Part model, mm, in its own coordinate system. A direction names the side the tool comes from. Round coordinates to 2 decimals unless told otherwise and drop trailing zeros. Write each loop counter-clockwise with the first axis right and the second up, starting at its lowest first coordinate (ties: lowest second). Pieces come first, ordered by that corner, then holes.
Autodesk Inventor part; units mm, degrees
ref_plane "YZ Plane" through (0, 0, 0) normal (1, 0, 0) x (0, 1, 0)
ref_plane "XZ Plane" through (0, 0, 0) normal (0, 1, 0) x (-1, 0, 0)
ref_plane "XY Plane" through (0, 0, 0) normal (0, 0, 1) x (1, 0, 0)
sketch "Sketch1" plane through (0, 0, 0) normal (1, 0, 0) x (0, 1, 0)
  line L0 (-81.3077, 45.4162) -> (50.6923, 45.4162)
  line L1 (56.553, 36.2588) -> (50.6923, 45.4162)
  line L2 (56.553, 36.2588) -> (63.703, 36.2588)
  line L3 (30.7678, 30.6662) -> (60.128, 30.6662)
  line L4 (63.703, 35.7588) -> (56.2794, 35.7588)
  line L5 (56.2794, 35.7588) -> (50.4187, 44.9162)
  line L6 (50.4187, 44.9162) -> (-81.3077, 44.9162)
  line L7 (63.703, 35.7588) -> (63.703, 36.2588)
  line L8 (-81.3077, 44.9162) -> (-81.3077, 45.4162)
  dimension "d26" = 132
  dimension "d29" = 7.15
  dimension "d31" = 0.5
  dimension "d38" = 29.5
revolve "Revolution1" add sketch "Sketch1" angle 360 about axis through (0, 30.7678, 30.6662) along (0, 1, 0)
sketch "Sketch2" plane through (0, -81.3077, 30.6662) normal (0, -1, 0) x (1, 0, 0)
  point P0 (0, -30.6662)
sketch "Sketch3" plane through (0, -81.3077, 30.6662) normal (0, -1, 0) x (1, 0, 0)
  line L0 (15, 15.5926) -> (-15, 15.5926)
  line L1 (-25, 5.5926) -> (-25, -5.5926)
  line L2 (-15, -15.5926) -> (15, -15.5926)
  line L3 (25, -5.5926) -> (25, 5.5926)
  arc A0 (-15, 15.5926) -> (-25, 5.5926) centre (-15, 5.5926) ccw
  arc A1 (-25, -5.5926) -> (-15, -15.5926) centre (-15, -5.5926) ccw
  arc A2 (15, -15.5926) -> (25, -5.5926) centre (15, -5.5926) ccw
  arc A3 (25, 5.5926) -> (15, 15.5926) centre (15, 5.5926) ccw
  circle A4 centre (0, 0) radius 14.25
  circle A5 centre (0, 0) radius 5.0926
  point P0 (0, -30.6662)
  point P1 (-25, -15.5926)
  point P2 (25, -15.5926)
  dimension "d34" = 50
  dimension "d35" = 10
extrude "Extrusion2" add sketch "Sketch3" along normal blind 2.37 contours A3 L3 A2 L2 A1 L1 A0 L0
properties part number "motor mount"
Q1. Wall check: line 1 (X direction, y = -70.5, z = 31.5); line 2 (X direction, y = -31, z = 39); line 3 (Y direction, x = 19, z = 35.5). Give the ranges that are in metal, low to high.
Q2. Saw through at B-B, the plane y = -71. Write the cut outline in (x, z).
Q3. Drop flat-ended pins along their axis: P1, Ø12, axis at x = -18, y = -51, coming from the -Z side; P2, Ø3, axis at x = 7.5, z = 39, coming from the +Y side; P3, Ø12, axis at x = -17.5, z = 18.5, coming from the +Y side. Give the stop position or say it passes through.
Q4. Tool access for faces 1 (the cylindrical face through (0.25, 60.18, 25.08)), 2 (the cylindrical face through (12.564, -15.691, 37.389)), 3 (the cylindrical face through (-21.993, -82.476, 17.925)): list every direction of +Z, -Z, +X, -X, +Y, -Y with a clear straight run to the whole face (end or side of a thin tool).
Q5. Saw through at A-A, the plane y = 53.5. Write the cut outline in (x, z), and give its area (3 significant figures).
Q6. Two-plate mould, pull along X, no slides. Class faces 4 (the cylindrical face through (-22.1, -82.5, 43.3)), 5 (the cylindrical face through (3.099, 59.939, 26.625)), 6 (the flat face through (5, 63.703, 29)): released by +X, released by -X, zero draft, split by the parting line, or undercut.
Computed:
1. line 1: x = -14.73 to -14.23, 14.23 to 14.73
1. line 2: x = -12.17 to -11.56, 11.56 to 12.17
1. line 3: y = -83.68 to -81.31
2. outline: circle Ø29.5 at (0, 30.67); hole circle Ø28.5 at (0, 30.67)
3. P1: stops at z = 22.09
3. P2: stops at y = 53.92
3. P3: stops at y = -81.31
4. face 1: +Y
4. face 2: -Y
4. face 3: -Z, -X, +Y, -Y
5. outline: circle Ø20.73 at (0, 30.67); hole circle Ø18.87 at (0, 30.67)
5. area: 57.7 mm2
6. face 4: released by -X
6. face 5: undercut
6. face 6: zero draft
